Source: CAD feature listing. Evaluate the final solid. Frame: model axes, mm. Face numbers are marked on the shaded views. A direction names the side the tool comes from. Give positions to 0.01 mm unless a question says otherwise; leave off trailing zeros. Order: outer loops, then holes, each group sorted by start corner. A loop starts at its lowest first (then second) coordinate and runs counter-clockwise, first axis right, second up. Notation, with made-up numbers: M 50,66.25 L 89,66.25 A19 ccw 89,97.25 Z; hole C 86,-36 d1. An arc over 180 degrees is marked long. Use CSV: the item, a comma, the result in double quotes. Start each with the question number.
Item 1: Section query A-A on z = 0. Return loops of the section in (x, y), and give its area (3 significant figures).
Item 2: Section query B-B on x = 3.65. Return loops of the section in (y, z), and give its area (3 significant figures).
Item 3: First-contact query: pin 1 (6 mm diameter, centred on y = 1.5, z = -5.5, fed in from -X); pin 2 (1.5 mm diameter, centred on x = 0.5, y = -1.5, fed in from +Z). Flat tips, straight axial feed; report the tip coordinate or a pass-through.
Item 4: Section query D-D on z = 3. Return loops of the section in (x, y), and give its area (3 significant figures).
Item 5: Ray query, probe 1 along Y at (x, z) = (-0.25, 0); probe 2 along Y at (x, z) = (1.35, 0); probe 3 along X at (y, z) = (4.5, -4). Return the intervals inside material, ascending. Write a range as from..to.
Item 6: Section query C-C on y = 0.25. Return loops of the section in (x, z), and give its area (3 significant figures).
Item 7: Access query for the marked faces 1 and 2. Directions: +Z, -Z, +X, -X, +Y, -Y. A direction counts if a zero-diameter tool reaches every point of the face in a straight line with its end or side. Return the directions, or none.
from build123d import *

# Parameters (mm, degrees)
SKETCH1_R           = 2.48
BOSS_EXTRUDE1_DEPTH = 4.572
SKETCH2_R           = 3.81
SKETCH2_R_2         = 2.48
BOSS_EXTRUDE2_DEPTH = 1.016


with BuildPart() as part:
    # Sketch1 → Boss-Extrude1 (new body)
    with BuildSketch(Plane(origin=(0, 0, 0), x_dir=(0, 0, -1), z_dir=(1, 0, 0))):
        Polygon((3.456884737, -5.9875), (6.913769474, 0), (3.456884737, 5.9875), (-3.456884737, 5.9875), (-6.913769474, 0), (-3.456884737, -5.9875), align=None)
        Circle(SKETCH1_R, mode=Mode.SUBTRACT)
    extrude(amount=BOSS_EXTRUDE1_DEPTH)

    # Sketch2 → Boss-Extrude2 (add)
    with BuildSketch(Plane(origin=(0, 0, 0), x_dir=(0, 0, -1), z_dir=(1, 0, 0))):
        Circle(SKETCH2_R)
        Circle(SKETCH2_R_2, mode=Mode.SUBTRACT)
    extrude(amount=-BOSS_EXTRUDE2_DEPTH)


solid = part.part
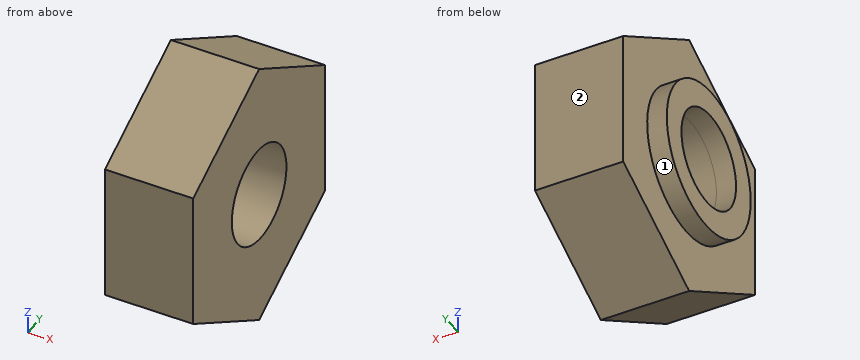
Verdict:
1,outline,"M -1.02,-3.81 L 0,-3.81 L 0,-5.99 L 4.57,-5.99 L 4.57,-2.48 L -1.02,-2.48 Z; M -1.02,2.48 L 4.57,2.48 L 4.57,5.99 L 0,5.99 L 0,3.81 L -1.02,3.81 Z"
1,area,"34.8 mm2"
2,outline,"M -5.99,-3.46 L 0,-6.91 L 5.99,-3.46 L 5.99,3.46 L 0,6.91 L -5.99,3.46 Z; hole C 0,0 d4.96"
2,area,"105 mm2"
3,pin 1,"x = -1.02"
3,pin 2,"z = 6.48"
4,outline,"M -1.02,-2.35 L 0,-2.35 L 0,-5.99 L 4.57,-5.99 L 4.57,5.99 L 0,5.99 L 0,2.35 L -1.02,2.35 Z"
4,area,"59.5 mm2"
5,probe 1,"-3.81..-2.48, 2.48..3.81"
5,probe 2,"-5.99..-2.48, 2.48..5.99"
5,probe 3,"0..4.57"
6,outline,"M -1.02,-3.8 L 0,-3.8 L 0,-6.77 L 4.57,-6.77 L 4.57,-2.47 L -1.02,-2.47 Z; M -1.02,2.47 L 4.57,2.47 L 4.57,6.77 L 0,6.77 L 0,3.8 L -1.02,3.8 Z"
6,area,"42.0 mm2"
7,face 1,"-X"
7,face 2,"+Z, -Z, +X, -X, +Y"
